The model under review builds one solid part; all positions refer to its coordinate system, in mm. A direction names the side the tool comes from. Round coordinates to 2 decimals unless told otherwise and drop trailing zeros. Order: outer loops, then holes, each group sorted by start corner. A loop starts at its lowest first (then second) coordinate and runs counter-clockwise, first axis right, second up.
from build123d import *

# Parameters (mm, degrees)
F1_DEPTH = 3


with BuildPart() as f1:
    # F0 (on Front) → F1 (new body)
    with BuildSketch(Plane.XZ):
        with BuildLine():
            Line((35, -1.5), (35, 1.5))
            Line((35, 1.5), (35, 5))
            Line((35, 5), (30, 5))
            Line((30, 5), (30, 2.95))
            Line((30, 2.95), (20.18628, 2.95))
            ThreePointArc((20.18628, 2.95), (17.692582, 1.86932), (15, 1.5))
            Line((15, 1.5), (-15, 1.5))
            ThreePointArc((-15, 1.5), (-17.692582, 1.86932), (-20.18628, 2.95))
            Line((-20.18628, 2.95), (-30, 2.95))
            Line((-30, 2.95), (-30, 5))
            Line((-30, 5), (-35, 5))
            Line((-35, 5), (-35, 1.5))
            Line((-35, 1.5), (-35, -1.5))
            Line((-35, -1.5), (-35, -5))
            Line((-35, -5), (-30, -5))
            Line((-30, -5), (-30, -2.95))
            Line((-30, -2.95), (-20.18628, -2.95))
            ThreePointArc((-20.18628, -2.95), (-17.692582, -1.86932), (-15, -1.5))
            Line((-15, -1.5), (15, -1.5))
            ThreePointArc((15, -1.5), (17.692582, -1.86932), (20.18628, -2.95))
            Line((20.18628, -2.95), (30, -2.95))
            Line((30, -2.95), (30, -5))
            Line((30, -5), (35, -5))
            Line((35, -5), (35, -1.5))
        make_face()
    extrude(amount=F1_DEPTH)


solid = f1.part
(1) Clearance check with flat-ended pins moving along their axes: P1, Ø1.5, axis at x = -26, y = -1, coming from the +Z side; P2, Ø1.5, axis at x = 9.5, z = 3, coming from the +Y side; P3, Ø0.9, axis at x = 24.5, y = -2, coming from the -Z side. State where each tip first meets the part, or that it passes through.
(2) We need section D-D (z = 2.25). Give the boundary of the cut face in (x, y).
(3) The part is to be moulded in two halves that separate along X. For faces 1 (the cylindrical face through (-17.66, -1.48, 1.86)), 2 (the flat face through (-30, -1, -4)), 3 (the flat face through (-35, -1, 0)), 4 (the flat face through (32, -1, -5)), say which applies: pulls with the +X half, pulls with the -X half, needs draft (parallel to the pull), parting line crosses it, or undercut.
(4) Tool access review of faces 5 (the flat face through (35, -1, 0)), 6 (the cylindrical face through (-17.73, -1.48, -1.88)), 7 (the flat face through (-25, -1, 2.95)): name each direction out of +Z, -Z, +X, -X, +Y, -Y from which nothing blocks a thin tool from reaching the whole face with its end or side.
(5) We need section C-C (x = -3.5). Give the boundary of the cut face in (y, z), and give its area (3 significant figures).
(6) We need section B-B (y = -1.25). Give the boundary of the cut face in (x, z).
(7) To check wall thickness, follow L1, parallel to X at y = -2.7, z = 4.25; L2, parallel to Z at x = -26.5, y = -1.7; L3, parallel to Z at x = -7, y = -0.8. State the ranges of each line that lie inside material, in increasing order.
(8) We need section A-A (z = -4.25). Give the boundary of the cut face in (x, y), and give its area (3 significant figures).
Verdict:
1. P1: stops at z = 2.95
1. P2: passes through
1. P3: stops at z = -2.95
2. outline: (-35, -3) - (-18.8, -3) - (-18.8, 0) - (-35, 0) - close; (18.8, -3) - (35, -3) - (35, 0) - (18.8, 0) - close
3. face 1: undercut
3. face 2: undercut
3. face 3: pulls with the -X half
3. face 4: needs draft
4. face 5: +Z, -Z, +X, +Y, -Y
4. face 6: -Z, +Y, -Y
4. face 7: +Z, +Y, -Y
5. outline: (-3, -1.5) - (0, -1.5) - (0, 1.5) - (-3, 1.5) - close
5. area: 9.00 mm2
6. outline: (-35, -5) - (-30, -5) - (-30, -2.95) - (-20.19, -2.95) arc R10 cw to (-15, -1.5) - (15, -1.5) arc R10 cw to (20.19, -2.95) - (30, -2.95) - (30, -5) - (35, -5) - (35, 5) - (30, 5) - (30, 2.95) - (20.19, 2.95) arc R10 cw to (15, 1.5) - (-15, 1.5) arc R10 cw to (-20.19, 2.95) - (-30, 2.95) - (-30, 5) - (-35, 5) - close
7. L1: x = -35 to -30, 30 to 35
7. L2: z = -2.95 to 2.95
7. L3: z = -1.5 to 1.5
8. outline: (-35, -3) - (-30, -3) - (-30, 0) - (-35, 0) - close; (30, -3) - (35, -3) - (35, 0) - (30, 0) - close
8. area: 30.0 mm2
